Autodesk Inventor part; units mm, degrees
ref_plane "YZ Plane" through (0, 0, 0) normal (1, 0, 0) x (0, 1, 0)
ref_plane "XZ Plane" through (0, 0, 0) normal (0, 1, 0) x (-1, 0, 0)
ref_plane "XY Plane" through (0, 0, 0) normal (0, 0, 1) x (1, 0, 0)
sketch "Sketch1" plane through (0, 0, 0) normal (0, 0, 1) x (1, 0, 0)
  line L0 (0, 0) -> (-10.3721, 0)
  line L1 (-10.3721, 0) -> (-10.3721, 14.357)
  line L2 (-10.3721, 14.357) -> (0, 14.357)
  line L3 (0, 14.357) -> (0, 0)
extrude "Extrusion1" add sketch "Sketch1" along normal blind 5
sketch "Sketch2" plane through (0, 0, 5) normal (0, 0, 1) x (1, 0, 0)
  line L0 (-8.8721, 12.857) -> (-1.5, 12.857)
  line L1 (-1.5, 12.857) -> (-1.5, 1.5)
  line L2 (-1.5, 1.5) -> (-8.8721, 1.5)
  line L3 (-8.8721, 1.5) -> (-8.8721, 12.857)
  line L4 (0, 14.357) -> (-10.3721, 14.357)
  line L5 (-10.3721, 0) -> (0, 0)
  line L6 (0, 0) -> (0, 14.357)
  line L7 (-10.3721, 14.357) -> (-10.3721, 0)
  dimension "d2" = 1.5
  dimension "d3" = 1.5
  dimension "d4" = 1.5
  dimension "d5" = 1.5
extrude "Extrusion2" cut sketch "Sketch2" against normal blind 2 contours L0 L1 L2 L3
sketch "Sketch3" plane through (0, 0, 3) normal (0, 0, 1) x (1, 0, 0)
  line L0 (-8.8721, 12.857) -> (-1.5, 12.857)
  line L1 (-8.8721, 1.5) -> (-8.8721, 12.857)
  line L2 (-1.5, 12.857) -> (-1.5, 1.5)
  line L3 (-1.5, 1.5) -> (-8.8721, 1.5)
  point P0 (0, 0)
fillet "Fillet1" radius 2 1 edges at (-10.3721, 14.357, 2.5)
fillet "Fillet2" radius 2 1 edges at (0, 14.357, 2.5)
fillet "Fillet3" radius 2 1 edges at (-10.3721, 0, 2.5)
fillet "Fillet4" radius 2 1 edges at (0, 0, 2.5)
sketch "Sketch4" plane through (-8.3721, 0, 0) normal (0, -1, 0) x (1, 0, 0)
  line L0 (6.3721, 0) -> (0, 0)
  ellipse E0 centre (3.186, 0) end of major axis (6.3721, 0) minor radius 1.4038
  point P0 (8.3721, 0)
extrude "Extrusion3" cut sketch "Sketch4" against normal blind 50
properties part number "bateria pat 1"
Source: CAD feature listing. Evaluate the final solid. Frame: model axes, mm. A direction names the side the tool comes from. Give positions to 0.01 mm unless a question says otherwise; leave off trailing zeros. Write each loop counter-clockwise with the first axis right and the second up, starting at its lowest first coordinate (ties: lowest second). Pieces come first, ordered by that corner, then holes. Notation, with made-up numbers: (14, 41.5) - (63, 41.5) arc R23 cw to (63, 66.5) - close; hole circle Ø4 at (-8, 48). An arc over 180 degrees is marked (long way). Write item = value, one per line. Start each with the question number.
Q1. Cut plane A-A, the plane z = 4.15. Return loops of the section in (x, y), then the cut area to 3 significant figures.
Q2. Material intervals for probe 1 along Y at (x, z) = (-2, 4.35); probe 2 along X at (y, z) = (6.5, 3.2); probe 3 along Z at (x, y) = (-5, 7), sorted ascending.
Q3. Cut plane B-B, the plane z = 2.3. Return loops of the section in (x, y), then the cut area to 3 significant figures.
Q4. Draft query along X for faces 1 (the flat face through (0, 7, 2)), 2 (the cylindrical face through (-9.8, 0.6, 2.5)), 3 (the flat face through (-1.5, 7, 4)). Return one class per face: +X half, -X half, draft (parallel to the pull), parting line (faces both ways), or undercut.
Q5. Pin query (flat end, axial travel): pin 1 Ø3 at (x, y) = (-3.5, 7) entering from +Z. Return the tip coordinate at first contact, or that it passes through.
Q6. Reachability of faces 4 (the flat face through (-5, 1.5, 4)), 5 (the flat face through (-1, 7, 0)) from +Z, -Z, +X, -X, +Y, -Y: full face, straight path, thin tool, end or side. Return the list, or none.
Computed values:
q1.outline = (-10.37, 2) arc R2 ccw to (-8.37, 0) - (-2, 0) arc R2 ccw to (0, 2) - (0, 12.36) arc R2 ccw to (-2, 14.36) - (-8.37, 14.36) arc R2 ccw to (-10.37, 12.36) - close; hole (-8.87, 1.5) - (-1.5, 1.5) - (-1.5, 12.86) - (-8.87, 12.86) - close
q1.area = 61.8 mm²
q2.probe_1 = 0 to 1.5, 12.86 to 14.36
q2.probe_2 = -10.37 to -8.87, -1.5 to 0
q2.probe_3 = 1.4 to 3
q3.outline = (-10.37, 2) arc R2 ccw to (-8.37, 0) - (-2, 0) arc R2 ccw to (0, 2) - (0, 12.36) arc R2 ccw to (-2, 14.36) - (-8.37, 14.36) arc R2 ccw to (-10.37, 12.36) - close
q3.area = 145 mm²
q4.face_1 = +X half
q4.face_2 = -X half
q4.face_3 = undercut
q5.pin_1 = 3
q6.face_4 = +Z
q6.face_5 = -Z, +X, -X, +Y, -Y
